Verification items for the finished model (mm, model axes). A direction names the side the tool comes from. Give positions to 0.01 mm unless a question says otherwise; leave off trailing zeros. Order: outer loops, then holes, each group sorted by start corner. A loop starts at its lowest first (then second) coordinate and runs counter-clockwise, first axis right, second up. Notation, with made-up numbers: (49, 2.5) -> (73, 2.5) arc R13 cw to (73, 15.5) -> close; hole circle Ø3 at (-20.5, 78.5). An arc over 180 degrees is marked (long way). Return JSON: item names as keys, results as strings. Group by question number.
(1) Cross-section at A-A on z = 0. Enter the section's corners in (x, y).
(2) Cross-section at C-C on x = -0.75. Enter the section's corners in (y, z), then the cut area to 3 significant figures.
(3) Thickness scan on line 1 along Y through (x, z) = (5.25, 0); line 2 along X through (y, z) = (0.75, -7.5); line 3 along Z through (x, y) = (-3.75, 1). Record the ranges inside material, lowest first.
(4) Tool access check on faces 1 (the face through (11, 2, -2)), 2 (the face through (5, 4.3, 0.1)). Record the directions out of +Z, -Z, +X, -X, +Y, -Y that give a thin tool (end or side, any length) a straight path to the whole face; none if there is none.
(5) Depth check by flat-ended pin: pin 1 Ø3 at (x, z) = (1, -9) entering from -Y; pin 2 Ø1.5 at (x, z) = (1, -5) entering from -Y; pin 3 Ø1.5 at (x, y) = (8.5, -0.5) entering from -Z. Enter the tip coordinate at first touch or a pass-through.
(6) Release check for a two-part mould opening along Z. For faces 3 (the face through (-5, 2, -2)), 4 (the face through (0.04, -11.99, 0.53)), 5 (the face through (2.89, 2.44, 0.54)) record: pulls with the +Z half, pulls with the -Z half, needs draft (parallel to the pull), parting line crosses it, or undercut.
(7) Cross-section at D-D on x = 3.5. Enter the section's corners in (y, z), then the cut area to 3 significant figures.
Autodesk Inventor part; units mm, degrees
ref_plane "YZ Plane" through (0, 0, 0) normal (1, 0, 0) x (0, 1, 0)
ref_plane "XZ Plane" through (0, 0, 0) normal (0, 1, 0) x (-1, 0, 0)
ref_plane "XY Plane" through (0, 0, 0) normal (0, 0, 1) x (1, 0, 0)
sketch "Sketch1" plane through (0, 0, 0) normal (0, 0, 1) x (1, 0, 0)
  line L0 (-5, 0) -> (5, 0)
  line L1 (-5, 0) -> (-5, 10)
  line L2 (-5, 10) -> (-3, 12)
  line L3 (-3, 12) -> (3, 12)
  line L4 (3, 12) -> (5, 10)
  line L5 (5, 10) -> (5, 0)
  point P0 (0, 0)
  point P1 (0, 0)
  point P2 (0, 12)
  dimension "d0" = 10
  dimension "d1" = 24
  dimension "d2" = 6
  dimension "d3" = 20
revolve "Revolution1" add sketch "Sketch1" angle 360 about axis through (-5, 0, 0) along (1, 0, 0)
sketch "Sketch2" plane through (5, 0, 0) normal (1, 0, 0) x (0, 0, -1)
  circle A0 centre (0, 0) radius 2.5
  dimension "d5" = 5
extrude "Extrusion1" cut sketch "Sketch2" against normal through all
sketch "Sketch3" plane through (5, 0, 0) normal (1, 0, 0) x (0, 0, -1)
  circle A0 centre (0, 0) radius 4
  circle A1 centre (0, 0) radius 2.5
  dimension "d8" = 8
extrude "Extrusion2" add sketch "Sketch3" along normal blind 6
properties part number "wheel"
Verdict:
{
 "1": {"outline": "(-5, -10) -> (-3, -12) -> (3, -12) -> (5, -10) -> (5, -4) -> (11, -4) -> (11, -2.5) -> (-5, -2.5) -> close; (-5, 2.5) -> (11, 2.5) -> (11, 4) -> (5, 4) -> (5, 10) -> (3, 12) -> (-3, 12) -> (-5, 10) -> close"},
 "2": {"outline": "circle Ø24 at (0, 0); hole circle Ø5 at (0, 0)", "area": "433 mm²"},
 "3": {"line 1": "-4 to -2.5, 2.5 to 4", "line 2": "-5 to 5", "line 3": "-11.21 to -2.29, 2.29 to 11.21"},
 "4": {"face 1": "+Z, -Z, +X, +Y, -Y", "face 2": "+X"},
 "5": {"pin 1": "y = -9.37", "pin 2": "y = -11.22", "pin 3": "z = -4"},
 "6": {"face 3": "needs draft", "face 4": "parting line crosses it", "face 5": "undercut"},
 "7": {"outline": "circle Ø23 at (0, 0); hole circle Ø5 at (0, 0)", "area": "396 mm²"}
}
